from build123d import *

# Parameters (mm, degrees)
SKETCH1_R           = 3.325
SKETCH1_W           = 3.575
SKETCH1_H           = 3.575
BOSS_EXTRUDE1_DEPTH = 6.35
CHAMFER1_SIZE       = 0.4
CHAMFER2_SIZE       = 0.2


with BuildPart() as part:
    # Sketch1 → Boss-Extrude1 (new body)
    with BuildSketch(Plane.XY):
        Circle(SKETCH1_R)
        Rectangle(SKETCH1_W, SKETCH1_H, mode=Mode.SUBTRACT)
    extrude(amount=BOSS_EXTRUDE1_DEPTH)

    # Chamfer1
    chamfer1_edges = [part.edges().sort_by_distance(p)[0] for p in [
        (-3.325, 0, 0),
        (-3.325, 0, 6.35),
    ]]
    chamfer(chamfer1_edges, length=CHAMFER1_SIZE)

    # Chamfer2
    chamfer2_edges = [part.edges().sort_by_distance(p)[0] for p in [
        (0, -1.7875, 6.35),
        (1.7875, 0, 0),
        (0, 1.7875, 0),
        (-1.7875, 0, 0),
        (0, -1.7875, 0),
        (1.7875, 0, 6.35),
        (0, 1.7875, 6.35),
        (-1.7875, 0, 6.35),
    ]]
    chamfer(chamfer2_edges, length=CHAMFER2_SIZE)


solid = part.part
Work out the finished part from the listing and answer in its coordinate system (mm). A direction names the side the tool comes from. Give positions to 0.01 mm unless a question says otherwise; leave off trailing zeros. Answer as a JSON object with one key per item and string values. Group by question number.
1. A flat-ended cylindrical pin translates along its axis: pin 1 Ø1 at (y, z) = (2, 1.5) entering from +X. Find the tip coordinate at first contact, or state that the pin passes through.
2. The mould has two halves that part along Y. Classify faces 3 (the flat face through (0, 1.788, 3)), 4 (the flat face through (0.2, -2.2, 6.35)), 5 (the cylindrical face through (1.53, -2.95, 3.14)), 6 (the flat face through (0, -1.788, 3)): released by +Y, released by -Y, zero draft, split by the parting line, or undercut.
3. A tool of negligible diameter and unlimited length cuts with its end or side. For faces 1 (the flat face through (0.2, -2.2, 0)), 2 (the flat face through (1.788, 0, 3)), from which of +Z, -Z, +X, -X, +Y, -Y can it reach the whole face along a straight path? Write none if from no direction.
4. Consider line 1 along Y through (x, z) = (0, 4) (1 decimal); line 2 along Y through (x, z) = (1.75, 3); line 3 along X through (y, z) = (0.25, 4). Determine where each line is inside the solid, lowest interval first. Write a range as [from, to].
Result sheet:
{
 "1": {"pin 1": "stops at x = 2.97"},
 "2": {"face 3": "undercut", "face 4": "zero draft", "face 5": "split by the parting line", "face 6": "undercut"},
 "3": {"face 1": "-Z, +X, -X, +Y, -Y", "face 2": "+Z, -Z"},
 "4": {"line 1": "y = [-3.3, -1.8], [1.8, 3.3]", "line 2": "y = [-2.83, -1.79], [1.79, 2.83]", "line 3": "x = [-3.32, -1.79], [1.79, 3.32]"}
}
